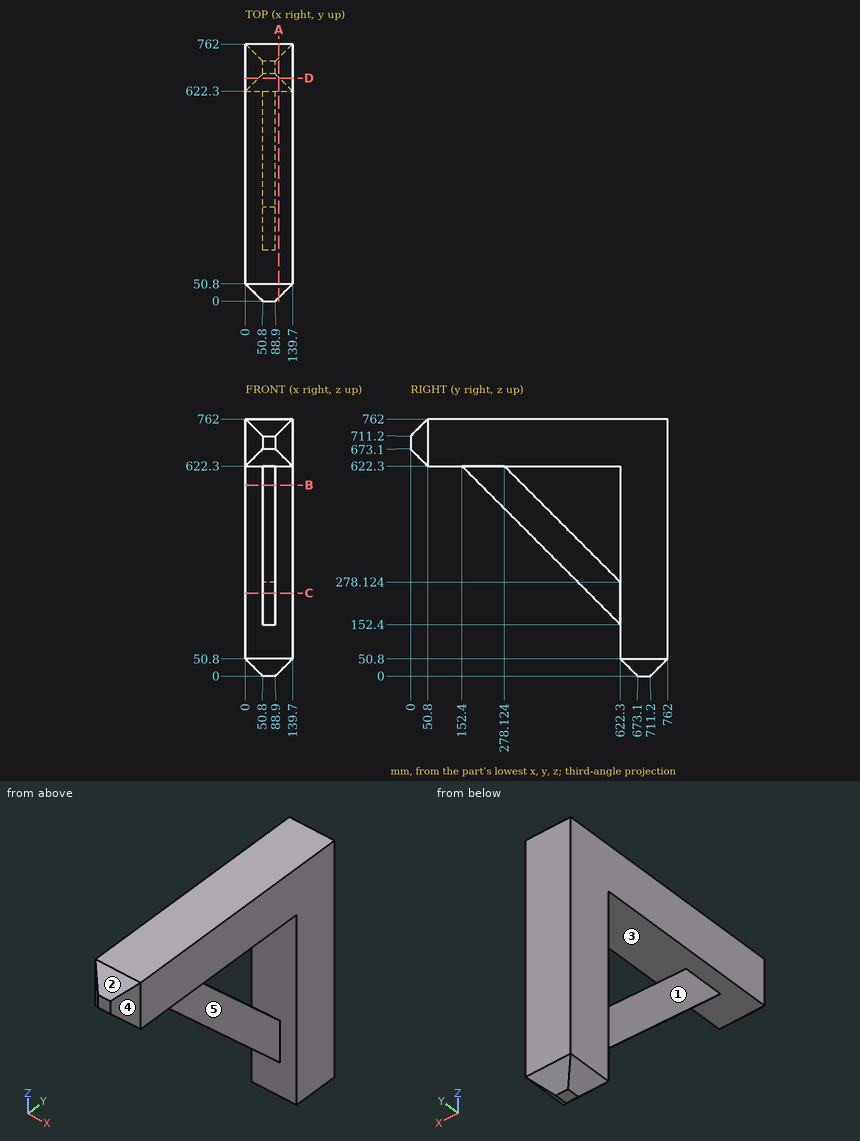
Could you check a few things on this drawing? It's one solid part, dimensions in mm from its lowest x, y, z. A direction names the side the tool comes from. Coordinates: 2 decimals unless noted, no trailing zeros. Write each loop counter-clockwise with the first axis right and the second up, starting at its lowest first coordinate (ties: lowest second). Pieces come first, ordered by that corner, then holes.
Q1. Imagine slicing it at C-C, the plane z = 245.5. List the corners of the cut face in (x, y) for me, plus the area to 3 significant figures.
Results found:
outline: (0, 622.3) - (50.8, 622.3) - (50.8, 529.2) - (88.9, 529.2) - (88.9, 622.3) - (139.7, 622.3) - (139.7, 762) - (0, 762) - close
area: 23,100 mm2
Q2. Imagine slicing it at D-D, the plane y = 661. List the corners of the cut face in (x, z) for me, plus the area to 3 significant figures.
Results found:
outline: (0, 50.8) - (38.7, 12.1) - (101, 12.1) - (139.7, 50.8) - (139.7, 762) - (0, 762) - close
area: 103,000 mm2
Q3. Imagine slicing it at A-A, the plane x = 99. List the corners of the cut face in (y, z) for me, plus the area to 3 significant figures.
Results found:
outline: (10.1, 663) - (50.8, 622.3) - (622.3, 622.3) - (622.3, 50.8) - (663, 10.1) - (721.3, 10.1) - (762, 50.8) - (762, 762) - (50.8, 762) - (10.1, 721.3) - close
area: 187,000 mm2
Q4. If we mould it in two halves opening along Y, with no side actions, what happens to the marked faces 1, 2 and 3? For each: +Y half, -Y half, draft (parallel to the pull), parting line (faces both ways), or undercut.
Results found:
face 1: draft
face 2: -Y half
face 3: undercut
Q5. Imagine slicing it at B-B, the plane z = 566. List the corners of the cut face in (x, y) for me, plus the area to 3 significant figures.
Results found:
outline: (0, 622.3) - (139.7, 622.3) - (139.7, 762) - (0, 762) - close; (50.8, 208.7) - (88.9, 208.7) - (88.9, 334.42) - (50.8, 334.42) - close
area: 24,300 mm2
Q6. Please list where these lines run through material, in increasing order: L1, parallel to Y at x = 18, z = 437.5; L2, parallel to X at y = 292, z = 484.5.
Results found:
L1: y = 622.3 to 762
L2: x = 50.8 to 88.9
Q7. Which directions (+Z, -Z, +X, -X, +Y, -Y) give clear straight access to the entire face, cutting with the end or side of a thin tool? Please do the marked faces 4 and 5.
Results found:
face 4: +Z, -Z, +X, -Y
face 5: -Z, +X, -Y
Q8. For P1, Ø8, axis at x = 18.5, y = 211, coming from the -Z side; P2, Ø10, axis at x = 58.5, y = 522, coming from the -Z side; P3, Ø8, axis at x = 123.5, z = 424.5, coming from the -Y side, each with a flat end and sliding along its axis, tell me the tip position at first contact or that it passes through.
Results found:
P1: stops at z = 622.3
P2: stops at z = 247.7
P3: stops at y = 622.3
